from build123d import *

# Parameters (mm, degrees)
SKETCH1_R           = 2.2
BOSS_EXTRUDE1_DEPTH = 5
SKETCH2_R           = 6.5
SKETCH2_R_2         = 2.2
BOSS_EXTRUDE2_DEPTH = 3


with BuildPart() as part:
    # Sketch1 → Boss-Extrude1 (new body)
    with BuildSketch(Plane(origin=(0, 0, 0), x_dir=(1, 0, 0), z_dir=(0, 1, 0))):
        with BuildLine():
            Line((-13.158208581, -1.850148868), (-21.850124899, 21.590213559))
            ThreePointArc((-21.850124899, 21.590213559), (-18.015528911, 29.944606033), (-9.661136437, 26.110010045))
            Line((-9.661136437, 26.110010045), (-0.969220119, 2.669647618))
            ThreePointArc((-0.969220119, 2.669647618), (-4.803816107, -5.684744856), (-13.158208581, -1.850148868))
        make_face()
        with Locations(Location((-7.06371435, 0.409749375, 0), (0, 0, 270))):  # turned: the seam where the file's is
            Circle(SKETCH1_R, mode=Mode.SUBTRACT)
        with BuildLine():
            Line((-13.692878775, 24.615000438), (-10.216112247, 15.238855467))
            ThreePointArc((-10.216112247, 15.238855467), (-11.513975505, 12.411214938), (-14.341616034, 13.709078195))
            Line((-14.341616034, 13.709078195), (-17.818382562, 23.085223166))
            ThreePointArc((-17.818382562, 23.085223166), (-16.520519304, 25.912863695), (-13.692878775, 24.615000438))
        make_face(mode=Mode.SUBTRACT)
    extrude(amount=BOSS_EXTRUDE1_DEPTH)

    # Sketch2 → Boss-Extrude2 (add)
    with BuildSketch(Plane(origin=(0, 5, 0), x_dir=(-1, 0, 0), z_dir=(0, 1, 0))):
        with Locations(Location((7.06371435, -0.409749375, 0), (0, 0, 200.345274498))):  # turned: the seam where the file's is
            Circle(SKETCH2_R)
        with Locations(Location((7.06371435, -0.409749375, 0), (0, 0, 90))):  # turned: the seam where the file's is
            Circle(SKETCH2_R_2, mode=Mode.SUBTRACT)
    extrude(amount=BOSS_EXTRUDE2_DEPTH)


solid = part.part
Input: part model. Units: mm. Frame: model coordinates. A direction names the side the tool comes from. Give positions to 0.01 mm unless a question says otherwise; leave off trailing zeros. Write each loop counter-clockwise with the first axis right and the second up, starting at its lowest first coordinate (ties: lowest second). Pieces come first, ordered by that corner, then holes. Notation, with made-up numbers: (65, 58.25) -> (107, 58.25) arc R21 ccw to (107, 70.25) -> close; hole circle Ø7 at (20, 81.5). An arc over 180 degrees is marked (long way). Use one line per item in the form item = value. Start each with the question number.
1) Ray query, probe 1 along Z at (x, y) = (-6, 6); probe 2 along Y at (x, z) = (-15, -7.5); probe 3 along X at (y, z) = (4, 0). Return the intervals inside material, ascending. Write a range as from..to.
2) Set-up query: faces 1 (the flat face through (-16.056, 2.465, -18.332)), 2 (the flat face through (-6, 8, 2)). Return all of +Z, -Z, +X, -X, +Y, -Y with unobstructed straight access to the full face (end or side cutting, diameter ignored); none if empty.
3) Section query D-D on x = -4.5. Return the cut outline in (y, z).
4) Section query C-C on y = 4.5. Return the cut outline in (x, z) (3 decimals).
5) Draft query along X for faces 3 (the cylindrical face through (-18.149, 2.465, -29.893)), 4 (the cylindrical face through (-6.403, 3.944, 1.689)), 5 (the cylindrical face through (-16.566, 2.465, -25.896)), 6 (the flat face through (-11, 0, -12)). Return one class per face: pulls with the +X half, pulls with the -X half, needs draft (parallel to the pull), parting line crosses it, or undercut.
6) Section query B-B on x = -7.5. Return the cut outline in (y, z).
7) Section query A-A on z = 1. Return the cut outline in (x, y), then the cut area to 3 significant figures.
8) Pin query (flat end, axial travel): pin 1 (1.5 mm diameter, centred on x = -16.5, y = 7, fed in from +Z); pin 2 (6 mm diameter, centred on x = -9, z = -10, fed in from +Y); pin 3 (1 mm diameter, centred on x = -3.5, y = 6, fed in from -Z). Return the tip coordinate at first contact, or that it passes through.
Outcome:
q1.probe_1 = -6.82..-2.34, 1.52..6
q1.probe_2 = 0..5
q1.probe_3 = -13.84..-9.23, -4.9..-0.58
q2.face_1 = +Y, -Y
q2.face_2 = +Z, -Z, +X, -X, +Y
q3.outline = (0, -12.19) -> (5, -12.19) -> (5, -6.38) -> (8, -6.38) -> (8, 5.56) -> (0, 5.56) -> close
q4.outline = (-21.85, -21.59) arc R6.5 ccw to (-9.661, -26.11) -> (-0.969, -2.67) arc R6.5 ccw to (-13.158, 1.85) -> close; hole (-17.818, -23.085) arc R2.2 ccw to (-13.693, -24.615) -> (-10.216, -15.239) arc R2.2 ccw to (-14.342, -13.709) -> close; hole circle Ø4.4 at (-7.064, -0.41)
q5.face_3 = parting line crosses it
q5.face_4 = undercut
q5.face_5 = undercut
q5.face_6 = needs draft
q6.outline = (0, -20.28) -> (5, -20.28) -> (5, -6.9) -> (8, -6.9) -> (8, -2.57) -> (0, -2.57) -> close; (0, 1.75) -> (8, 1.75) -> (8, 6.08) -> (0, 6.08) -> close
q7.outline = (-13.47, 0) -> (-8.75, 0) -> (-8.75, 8) -> (-13.41, 8) -> (-13.41, 5) -> (-13.47, 5) -> close; (-5.37, 0) -> (-0.72, 0) -> (-0.72, 8) -> (-5.37, 8) -> close
q7.area = 74.8 mm^2
q8.pin_1 = through
q8.pin_2 = 5
q8.pin_3 = -6.14
